```python
from build123d import *

# Parameters (mm, degrees)
BASE_FLANGE1_DEPTH      = 62
CUT_EXTRUDE4_START      = -23
CUT_EXTRUDE4_OUTLINE_R  = 1.3
CUT_EXTRUDE4_DEPTH      = 46
CUT_EXTRUDE5_DEPTH      = 69.804069647
CUT_EXTRUDE5_DEPTH_BACK = 69.804069647
SKETCH9_W               = 9
SKETCH9_H               = 7.5
CUT_EXTRUDE7_DEPTH      = 69.804069647
CUT_EXTRUDE7_DEPTH_BACK = 69.804069647
SKETCH12_W              = 5.5
SKETCH12_H              = 26
SKETCH14_W              = 5
SKETCH14_H              = 11
CUT_EXTRUDE8_DEPTH      = 18
FILLET1_R               = 10
FILLET2_R               = 2
FILLET3_R               = 1


# Read off the part's stored shape, not the designer's step: Cut-Extrude4
# Sheet-metal steps are written as plain solids
with BuildPart() as part:
    # Sketch2 → Base-Flange1 (new body)
    with BuildSketch(Plane(origin=(0, 0, 0), x_dir=(1, 0, 0), z_dir=(0, 1, 0))):
        with BuildLine():
            Line((-21.5, 19), (-21.5, 2.5))
            ThreePointArc((-21.5, 2.5), (-20.767766953, 0.732233047), (-19, 0))
            Line((-19, 0), (19, 0))
            ThreePointArc((19, 0), (20.767766953, 0.732233047), (21.5, 2.5))
            Line((21.5, 2.5), (21.5, 19))
            Line((21.5, 19), (23, 19))
            Line((23, 19), (23, 2.5))
            ThreePointArc((23, 2.5), (21.828427125, -0.328427125), (19, -1.5))
            Line((19, -1.5), (-19, -1.5))
            ThreePointArc((-19, -1.5), (-21.828427125, -0.328427125), (-23, 2.5))
            Line((-23, 2.5), (-23, 19))
            Line((-23, 19), (-21.5, 19))
        make_face()
    extrude(amount=BASE_FLANGE1_DEPTH)

    # Cut-Extrude4 outline → Cut-Extrude4 (cut)
    with BuildSketch(Plane(origin=(0, 0, 0), x_dir=(0, 0, -1), z_dir=(1, 0, 0)).offset(CUT_EXTRUDE4_START)):
        with Locations((15.5, 2.5)):
            Circle(CUT_EXTRUDE4_OUTLINE_R)
        with Locations((13.156854249, 8.156854249)):
            Circle(CUT_EXTRUDE4_OUTLINE_R)
        with Locations((7.5, 10.5)):
            Circle(CUT_EXTRUDE4_OUTLINE_R)
        with BuildLine():
            ThreePointArc((12.5, 2.5), (7.5, 7.5), (2.5, 2.5))
            Line((2.5, 2.5), (2.5, 0))
            Line((2.5, 0), (12.5, 0))
            Line((12.5, 0), (12.5, 2.5))
        make_face()
    extrude(amount=CUT_EXTRUDE4_DEPTH, mode=Mode.SUBTRACT)

    # Sketch9 → Cut-Extrude5 (cut, two sides: drawn at the far end of the back side and taken through both)
    with BuildSketch(Plane(origin=(0, 0, 0), x_dir=(0, 0, -1), z_dir=(1, 0, 0)).offset(-CUT_EXTRUDE5_DEPTH_BACK)):
        with Locations((3, 3.75)):
            Rectangle(SKETCH9_W, SKETCH9_H)
    extrude(amount=CUT_EXTRUDE5_DEPTH + CUT_EXTRUDE5_DEPTH_BACK, mode=Mode.SUBTRACT)

    # Sketch12 → Cut-Extrude7 (cut, two sides: drawn at the far end of the back side and taken through both)
    with BuildSketch(Plane(origin=(0, 0, 0), x_dir=(0, 0, -1), z_dir=(1, 0, 0)).offset(-CUT_EXTRUDE7_DEPTH_BACK)):
        with Locations((1.25, 20.5)):
            Rectangle(SKETCH12_W, SKETCH12_H)
    extrude(amount=CUT_EXTRUDE7_DEPTH + CUT_EXTRUDE7_DEPTH_BACK, mode=Mode.SUBTRACT)

    # Sketch14 → Cut-Extrude8 (cut)
    with BuildSketch(Plane(origin=(23, 0, 0), x_dir=(0, 0, -1), z_dir=(1, 0, 0))):
        with Locations((1, 44)):
            Rectangle(SKETCH14_W, SKETCH14_H)
    extrude(amount=-CUT_EXTRUDE8_DEPTH, mode=Mode.SUBTRACT)

    # Fillet1
    fillet1_edges = [part.edges().sort_by_distance(p)[0] for p in [
        (-22.25, 62, -19),
        (22.25, 62, -19),
    ]]
    fillet(fillet1_edges, radius=FILLET1_R)

    # Fillet2
    fillet2_edges = [part.edges().sort_by_distance(p)[0] for p in [
        (-22.25, 0, -19),
        (22.25, 0, -19),
        (22.25, 7.5, -4),
        (-22.25, 7.5, -4),
        (5, 49.5, 0.75),
        (5, 38.5, 0.75),
        (-22.25, 0, -12.5),
        (22.25, 0, -12.5),
    ]]
    fillet(fillet2_edges, radius=FILLET2_R)

    # Fillet3
    fillet3_edges = [part.edges().sort_by_distance(p)[0] for p in [
        (22.25, 33.5, -4),
        (-22.25, 33.5, -4),
        (22.25, 49.5, -3.5),
        (22.25, 38.5, -3.5),
    ]]
    fillet(fillet3_edges, radius=FILLET3_R)


solid = part.part
```
Build history of the part. All positions in model axes, mm. A direction names the side the tool comes from. Round coordinates to 2 decimals unless told otherwise and drop trailing zeros. Order: outer loops, then holes, each group sorted by start corner. A loop starts at its lowest first (then second) coordinate and runs counter-clockwise, first axis right, second up. Notation, with made-up numbers: (-27, 69) -> (31, 69) arc R23 cw to (31, 101) -> close; hole circle Ø2 at (4, 27.5). An arc over 180 degrees is marked (long way). Answer in a Markdown table with one row per item.
1) Which spindle directions (+Z, -Z, +X, -X, +Y, -Y) get a long thin tool onto all of the face, cutting with end or side? Do faces 1 (the cylindrical face through (22.24, 6.888, -12.875)), 2 (the flat face through (-22, 27, -19)), 3 (the cylindrical face through (-21, 48, -1)), 4 (the flat face through (5, 44, 1)), 5 (the flat face through (22, 44, -3.5)). Say none if no direction does.
Values:
| item | result |
|---|---|
| face 1 | +X, -X |
| face 2 | -Z, +X, -X, +Y, -Y |
| face 3 | -Z, +Y, -Y |
| face 4 | +Z, -Z, +X |
| face 5 | +Z, +X |
2) Mould opens along Y. For faces 6 (the flat face through (-22, 21, -4)), 7 (the cylindrical face through (5.57, 48.9, 0.74)), 8 (the cylindrical face through (-22.24, 0.57, -13.1)) say: released by +Y, released by -Y, zero draft, split by the parting line, or undercut.
Values:
| item | result |
|---|---|
| face 6 | zero draft |
| face 7 | undercut |
| face 8 | released by -Y |
3) Band-saw the part on A-A on x = 12. Give the cut face in (y, z).
Values:
| item | result |
|---|---|
| outline | (33.5, 0) -> (38.5, 0) -> (38.5, 1.5) -> (33.5, 1.5) -> close; (49.5, 0) -> (62, 0) -> (62, 1.5) -> (49.5, 1.5) -> close |
4) Band-saw the part on D-D on x = -4.5. Give the cut face in (y, z).
Values:
| item | result |
|---|---|
| outline | (33.5, 0) -> (62, 0) -> (62, 1.5) -> (33.5, 1.5) -> close |
5) Wall check: L1, parallel to X at y = 55.5, z = -6.5; L2, parallel to Z at x = 22.2, y = 10.5; L3, parallel to Z at x = -22.1, y = 2.5. Give the ranges that are in metal, low to high.
Values:
| item | result |
|---|---|
| L1 | -23 to -21.5, 21.5 to 23 |
| L2 | -19 to -8.8, -6.2 to -4 |
| L3 | -19 to -16.8, -14.2 to -12.5 |
6) Band-saw the part on C-C on z = -15.5. Give the cut face in (x, y), and give its area (3 significant figures).
Values:
| item | result |
|---|---|
| outline | (-23, 0) -> (-21.5, 0) -> (-21.5, 1.2) -> (-23, 1.2) -> close; (-23, 3.8) -> (-21.5, 3.8) -> (-21.5, 59.6) -> (-23, 59.6) -> close; (21.5, 0) -> (23, 0) -> (23, 1.2) -> (21.5, 1.2) -> close; (21.5, 3.8) -> (23, 3.8) -> (23, 59.6) -> (21.5, 59.6) -> close |
| area | 171 mm2 |
7) Band-saw the part on B-B on y = 10.5. Give the cut face in (x, z).
Values:
| item | result |
|---|---|
| outline | (-23, -19) -> (-21.5, -19) -> (-21.5, -8.8) -> (-23, -8.8) -> close; (-23, -6.2) -> (-21.5, -6.2) -> (-21.5, -4) -> (-23, -4) -> close; (21.5, -19) -> (23, -19) -> (23, -8.8) -> (21.5, -8.8) -> close; (21.5, -6.2) -> (23, -6.2) -> (23, -4) -> (21.5, -4) -> close |
8) Pin check, flat tips, straight feed: P1, Ø0.8, axis at y = 43, z = 1, coming from the +X side; P2, Ø2.5, axis at y = 8.16, z = -13.16, coming from the -X side; P3, Ø14, axis at x = -6.5, y = 44, coming from the -Z side; P4, Ø0.8, axis at x = 22.5, y = 44.5, coming from the +Z side. Stop position of each tip, or through.
Values:
| item | result |
|---|---|
| P1 | x = 5 |
| P2 | through |
| P3 | z = 0 |
| P4 | z = -3.5 |
